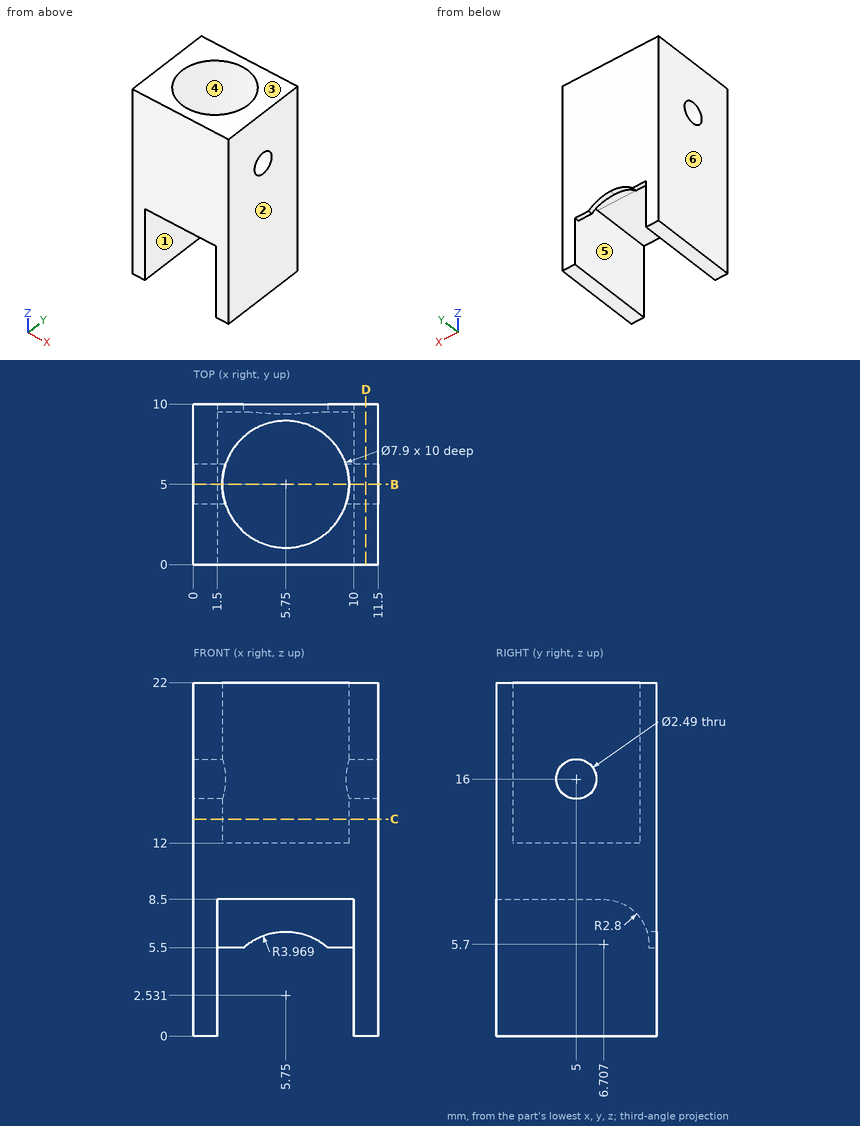
Here's the drawing with two shaded views (mm, measured from the low corner). I have some questions. A direction names the side the tool comes from. Round coordinates to 2 decimals unless told otherwise and drop trailing zeros. Order: outer loops, then holes, each group sorted by start corner. A loop starts at its lowest first (then second) coordinate and runs counter-clockwise, first axis right, second up. Notation, with made-up numbers: (-20, 18.5) -> (-10, 18.5) arc R22 ccw to (-10, 55.5) -> close; hole circle Ø7 at (41.5, 82). An arc over 180 degrees is marked (long way). Use a Markdown table: item, result. Add a question column.
(1) I need wall thicknesses on line 1 along Y through (x, z) = (10.25, 16) (1 decimal); line 2 along Z through (x, y) = (11, 5) (1 decimal); line 3 along X through (y, z) = (7.25, 3.75). Which ranges of each line are inside material? Lowest first, please.
(2) If we mould it in two halves opening along X, with no side actions, what happens to the marked faces 1, 2 and 3? For each: released by +X, released by -X, zero draft, split by the parting line, or undercut.
(3) Suppose I cut it at C-C, the plane z = 13.5. Please give me the cut outline in (x, y).
(4) For the marked faces 4, 5 and 6, which set-ups out of +Z, -Z, +X, -X, +Y, -Y let a thin tool reach every point of the face, with its end or its side?
(5) Suppose I cut it at B-B, the plane y = 5. Please give me the cut outline in (x, z) (1 decimal).
(6) Suppose I cut it at D-D, the plane x = 10.75. Please give me the cut outline in (y, z) (1 decimal).
(7) For pin 1 Ø5.5 at (x, y) = (6.5, 3) entering from -Z; pin 2 Ø4 at (x, y) = (4, 5.5) entering from +Z, each with a flat end and sliding along its axis, tell me the tip position at first contact or that it passes through.
Verdict:
| question | item | result |
|---|---|---|
| 1 | line 1 | 0 to 3.8, 6.2 to 10 |
| 1 | line 2 | 0 to 14.8, 17.2 to 22 |
| 1 | line 3 | 0 to 1.5, 10 to 11.5 |
| 2 | face 1 | undercut |
| 2 | face 2 | released by +X |
| 2 | face 3 | zero draft |
| 3 | outline | (0, 0) -> (11.5, 0) -> (11.5, 10) -> (0, 10) -> close; hole circle Ø7.9 at (5.75, 5) |
| 4 | face 4 | +Z |
| 4 | face 5 | -Z, -Y |
| 4 | face 6 | +Z, -Z, -X, +Y, -Y |
| 5 | outline | (0, 0) -> (1.5, 0) -> (1.5, 8.5) -> (10, 8.5) -> (10, 0) -> (11.5, 0) -> (11.5, 14.8) -> (9.7, 14.8) -> (9.7, 12) -> (1.8, 12) -> (1.8, 14.8) -> (0, 14.8) -> close; (0, 17.2) -> (1.8, 17.2) -> (1.8, 22) -> (0, 22) -> close; (9.7, 17.2) -> (11.5, 17.2) -> (11.5, 22) -> (9.7, 22) -> close |
| 6 | outline | (0, 0) -> (10, 0) -> (10, 22) -> (0, 22) -> close; hole circle Ø2.5 at (5, 16) |
| 7 | pin 1 | z = 8.5 |
| 7 | pin 2 | z = 12 |
